Verification items for this drawing (mm, ordinates from the low corner). A direction names the side the tool comes from. Give positions to 0.01 mm unless a question says otherwise; leave off trailing zeros. Write each loop counter-clockwise with the first axis right and the second up, starting at its lowest first coordinate (ties: lowest second). Pieces come first, ordered by that corner, then holes. Notation, with made-up numbers: (75.5, 56.5) -> (83.5, 56.5) arc R17 ccw to (83.5, 86.5) -> close; hole circle Ø11 at (67, 37). An arc over 180 degrees is marked (long way). Use one line per item in the form item = value. Start each with the question number.
(1) Release check for a two-part mould opening along X. For the marked faces 3, 4, 5 and 6 record: pulls with the +X half, pulls with the -X half, needs draft (parallel to the pull), parting line crosses it, or undercut.
(2) Section check A-A, the plane y = 4.5. Record the cut outline in (x, z), plus the area to 3 significant figures.
(3) Section check B-B, the plane x = 8. Record the cut outline in (y, z), plus the area to 3 significant figures.
(4) Section check D-D, the plane z = 16.5. Record the cut outline in (x, y).
(5) Set-up check for the marked faces 1 and 2: record each of +Z, -Z, +X, -X, +Y, -Y from which the full face is reachable in a straight line by a thin tool's end or side.
(6) Depth check by flat-ended pin: pin 1 Ø4 at (x, y) = (8, 4.5) entering from -Z; pin 2 Ø4 at (x, z) = (9.5, 9) entering from -Y; pin 3 Ø1.8 at (x, y) = (17, 4.5) entering from -Z. Enter the tip coordinate at first touch or a pass-through.
(7) Section check C-C, the plane y = 1.75. Record the cut outline in (x, z), plus the area to 3 significant figures.
(8) Scan lines: L1, parallel to Y at x = 17, z = 16.5; L2, parallel to Y at x = 9, z = 14; L3, parallel to Z at x = 2, y = 7. Record each from-to range of solid material in increasing order.
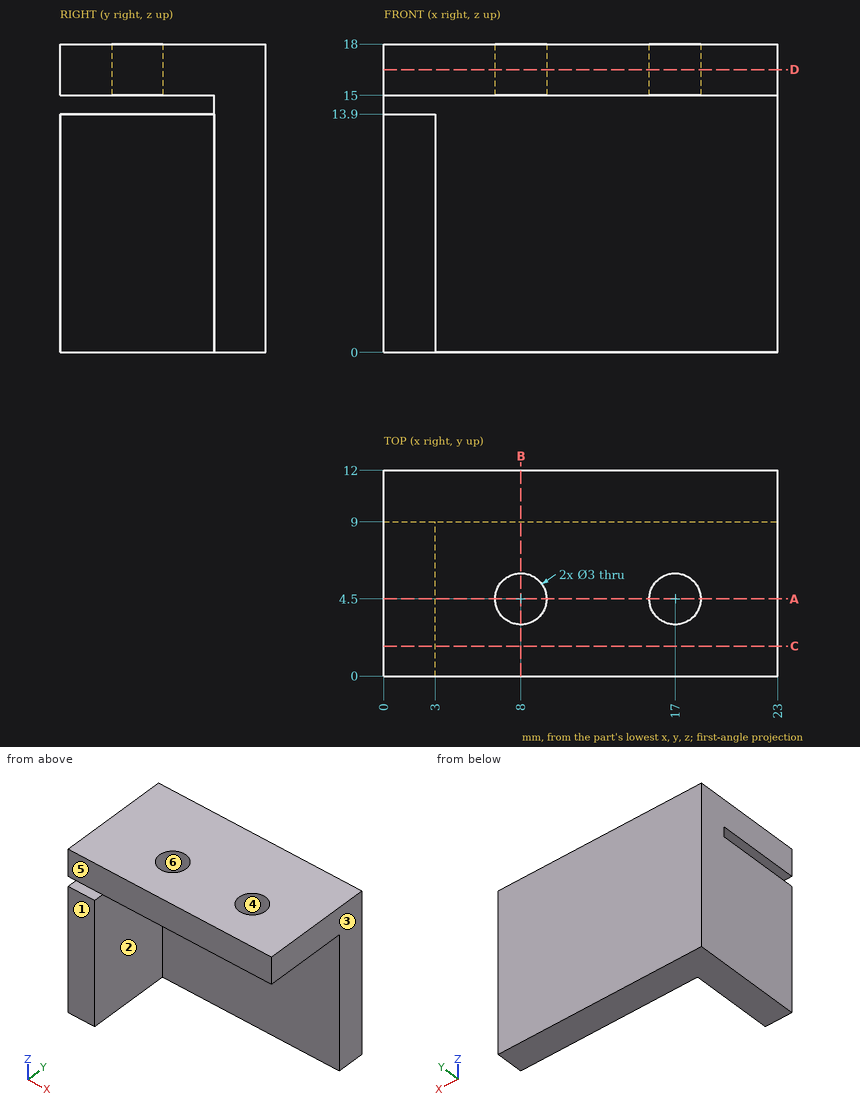
Completed:
q1.face_3 = pulls with the +X half
q1.face_4 = undercut
q1.face_5 = needs draft
q1.face_6 = undercut
q2.outline = (0, 0) -> (3, 0) -> (3, 13.9) -> (0, 13.9) -> close; (0, 15) -> (6.5, 15) -> (6.5, 18) -> (0, 18) -> close; (9.5, 15) -> (15.5, 15) -> (15.5, 18) -> (9.5, 18) -> close; (18.5, 15) -> (23, 15) -> (23, 18) -> (18.5, 18) -> close
q2.area = 92.7 mm²
q3.outline = (0, 15) -> (3, 15) -> (3, 18) -> (0, 18) -> close; (6, 15) -> (9, 15) -> (9, 0) -> (12, 0) -> (12, 18) -> (6, 18) -> close
q3.area = 72.0 mm²
q4.outline = (0, 0) -> (23, 0) -> (23, 12) -> (0, 12) -> close; hole circle Ø3 at (8, 4.5); hole circle Ø3 at (17, 4.5)
q5.face_1 = +Z, -Z, +X, -X, -Y
q5.face_2 = -Z, +X, -Y
q6.pin_1 = 15
q6.pin_2 = 9
q6.pin_3 = through
q7.outline = (0, 0) -> (3, 0) -> (3, 13.9) -> (0, 13.9) -> close; (0, 15) -> (23, 15) -> (23, 18) -> (0, 18) -> close
q7.area = 111 mm²
q8.L1 = 0 to 3, 6 to 12
q8.L2 = 9 to 12
q8.L3 = 0 to 13.9, 15 to 18
